Verification items for the finished model (mm, model axes). Face numbers are marked on the shaded views. Give positions to 0.01 mm unless a question says otherwise; leave off trailing zeros. Order: outer loops, then holes, each group sorted by start corner. A loop starts at its lowest first (then second) coordinate and runs counter-clockwise, first axis right, second up.
(1) Gauge pin test, flat end, axial feed: pin 1 (20.5 mm diameter, centred on y = -308, z = 31.5, fed in from -X) (3 decimals). Record the tip position at first contact, or that the pin passes through.
(2) Sectioned sample at B-B on x = 4.75. Record the cut outline in (y, z) (3 decimals), plus the area to 3 significant figures.
(3) Mould release check, pull along Z, two halves, no side actions. Record for the marked faces 1 and 2: pulls with the +Z half, pulls with the -Z half, needs draft (parallel to the pull), parting line crosses it, or undercut.
(4) Scan lines: L1, parallel to Z at x = 5, y = -143 (3 decimals); L2, parallel to Z at x = 10.2, y = -63.5; L3, parallel to Y at x = 11.75, z = 40.5. Record each from-to range of solid material in increasing order.
(5) Sectioned sample at C-C on z = 10.5. Record the cut outline in (x, y) (3 decimals).
```python
from build123d import *

# Parameters (mm, degrees)
F1_DEPTH = 457.2
F2_R     = 1.5875
F3_R     = 3.175
F4_R     = 7.14375
F4_R_2   = 19.84375
F4_R_3   = 7.9375
F5_DEPTH = 25.4


with BuildPart() as f1:
    # F0 (on Front) → F1 (new body)
    with BuildSketch(Plane.XZ):
        Polygon((0, 3.175), (0, 0), (12.7, 0), (12.7, 50.8), (0, 50.8), (0, 47.625), (9.525, 47.625), (9.525, 3.175), align=None)
    extrude(amount=F1_DEPTH)

    # F2
    f2_edges = [f1.edges().sort_by_distance(p)[0] for p in [
        (9.525, -228.6, 3.175),
        (9.525, -228.6, 47.625),
    ]]
    fillet(f2_edges, radius=F2_R)

    # F3
    f3_edges = [f1.edges().sort_by_distance(p)[0] for p in [
        (12.7, -228.6, 0),
        (12.7, -228.6, 50.8),
    ]]
    fillet(f3_edges, radius=F3_R)

    # F4 (on face) → F5 (cut)
    with BuildSketch(Plane.YZ.offset(12.7)):
        with Locations((-388.9375, 25.4)):
            Circle(F4_R)
        with Locations((-246.0625, 25.4)):
            Circle(F4_R)
        with Locations((-317.5, 25.4)):
            Circle(F4_R_2)
        with Locations((-63.5, 25.4)):
            Circle(F4_R_3)
    extrude(amount=-F5_DEPTH, mode=Mode.SUBTRACT)


solid = f1.part
```
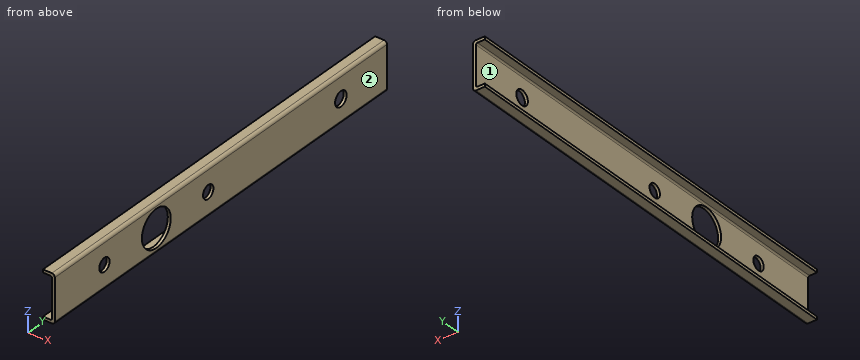
Ans:
1. pin 1: stops at x = 9.525
2. outline: (-457.2, 0) - (0, 0) - (0, 3.175) - (-457.2, 3.175) - close; (-457.2, 47.625) - (0, 47.625) - (0, 50.8) - (-457.2, 50.8) - close
2. area: 2,900 mm2
3. face 1: undercut
3. face 2: needs draft
4. L1: z = 0 to 3.175, 47.625 to 50.8
4. L2: z = 0.07 to 17.46, 33.34 to 50.73
4. L3: y = -457.2 to -330.37, -304.63 to 0
5. outline: (9.525, -457.2) - (12.7, -457.2) - (12.7, -330.606) - (9.525, -330.606) - close; (9.525, -304.394) - (12.7, -304.394) - (12.7, 0) - (9.525, 0) - close
